from build123d import *

# Parameters (mm, degrees)
M2_5X0_45_TAPPED_HOLE1_D     = 2.05
M2_5X0_45_TAPPED_HOLE1_DEPTH = 6.35
M2_5X0_45_TAPPED_HOLE1_TIP   = 0.615882135


with BuildPart() as part:
    # Sketch1 → Revolve1 (revolve)
    with BuildSketch(Plane.XY, mode=Mode.PRIVATE) as revolve1_sk:
        Polygon((0, 12.7), (-12.7, 12.7), (-12.7, 6.35), (-11.6205, 6.35), (-11.6205, -12.7), (0, -12.7), align=None)
    revolve(revolve1_sk.sketch.rotate(Axis((0, -12.7, 0), (0, 1, 0)), 180), axis=Axis((0, -12.7, 0), (0, 1, 0)))

    # M2.5x0.45 Tapped Hole1
    with Locations(Plane(origin=(0, 12.7, 0), x_dir=(1, 0, 0), z_dir=(0, 1, 0))):
        with Locations((0, 0)):
            Hole(M2_5X0_45_TAPPED_HOLE1_D / 2, depth=M2_5X0_45_TAPPED_HOLE1_DEPTH)
            with Locations((0, 0, -(M2_5X0_45_TAPPED_HOLE1_DEPTH + M2_5X0_45_TAPPED_HOLE1_TIP / 2))):  # 118° drill point
                Cone(0, M2_5X0_45_TAPPED_HOLE1_D / 2, M2_5X0_45_TAPPED_HOLE1_TIP, mode=Mode.SUBTRACT)


solid = part.part
Check sheet for the modelled part. Datum: model origin and axes. Units: mm. A direction names the side the tool comes from. Round coordinates to 2 decimals unless told otherwise and drop trailing zeros. Loops run counter-clockwise (first coordinate to the right, second up) from the corner with the lowest first, then second, coordinate; pieces in that order, holes last. Notation, with made-up numbers: M 49,50.5 L 59,50.5 A17 ccw 59,64.5 Z; hole C -24,-1 d6. An arc over 180 degrees is marked long. One line per question, with ' | ' between items. Start each with the question number.
Item 1: Set-up check for faces 4 (the face through (0.133, 9.481, -1.016)), 5 (the face through (-3, 12.7, 0)): record each of +Z, -Z, +X, -X, +Y, -Y from which the full face is reachable in a straight line by a thin tool's end or side.
Item 2: Scan lines: probe 1 along Z at (x, y) = (0, 8) (3 decimals); probe 2 along Y at (x, z) = (11.5, 3); probe 3 along Z at (x, y) = (0.25, -7). Record each from-to range of solid material in increasing order.
Item 3: Section check B-B (y = 10.75). Record the boundary of the cut face in (x, z) (3 decimals), and give its area (3 significant figures).
Item 4: Section check C-C (y = -7.5). Record the boundary of the cut face in (x, z).
Item 5: Gauge pin test, flat ends, axial feed: pin 1 Ø1.5 at (y, z) = (3.5, -1.5) entering from -X; pin 2 Ø8 at (y, z) = (7, -6) entering from -X; pin 3 Ø6 at (y, z) = (-9, -0.5) entering from +X; pin 4 Ø6 at (x, z) = (-10, 9) entering from -Y. Record the tip position at first contact, or that the pin passes through.
Item 6: Section check D-D (z = -6). Record the boundary of the cut face in (x, y), and give its area (3 significant figures).
Item 7: Release check for a two-part mould opening along Z. For faces 1 (the face through (-0.04, 5.84, 0.17)), 2 (the face through (-2.519, -3.308, 11.344)), 3 (the face through (11.2, 6.35, 3.7)) record: released by +Z, released by -Z, zero draft, split by the parting line, or undercut.
Item 8: Section check A-A (x = 8.25). Record the boundary of the cut face in (y, z), and give its area (3 significant figures).
Worked out:
1) face 4: +Y | face 5: +Z, -Z, +X, -X, +Y
2) probe 1: -12.7 to -1.025, 1.025 to 12.7 | probe 2: 6.35 to 12.7 | probe 3: -11.62 to 11.62
3) outline: C 0,0 d25.4; hole C 0,0 d2.05 | area: 503 mm^2
4) outline: C 0,0 d23.24
5) pin 1: x = -11.6 | pin 2: x = -12.54 | pin 3: x = 11.62 | pin 4: y = -12.7
6) outline: M -11.19,6.35 L -9.95,6.35 L -9.95,-12.7 L 9.95,-12.7 L 9.95,6.35 L 11.19,6.35 L 11.19,12.7 L -11.19,12.7 Z | area: 521 mm^2
7) face 1: undercut | face 2: split by the parting line | face 3: zero draft
8) outline: M -12.7,-8.18 L 6.35,-8.18 L 6.35,-9.66 L 12.7,-9.66 L 12.7,9.66 L 6.35,9.66 L 6.35,8.18 L -12.7,8.18 Z | area: 434 mm^2
